The listing builds one solid part. Answer for the finished solid, in the listing's coordinates (mm). Round coordinates to 2 decimals unless told otherwise and drop trailing zeros. Write each loop counter-clockwise with the first axis right and the second up, starting at its lowest first coordinate (ties: lowest second). Pieces come first, ordered by that corner, then holes.
from build123d import *

# Parameters (mm, degrees)
SKETCH1_R           = 5.2
SKETCH1_R_2         = 10
BOSS_EXTRUDE1_DEPTH = 6
BOSS_EXTRUDE2_DEPTH = 6
BOSS_EXTRUDE4_DEPTH = 6


with BuildPart() as part:
    # Sketch1 → Boss-Extrude1 (new body)
    with BuildSketch(Plane(origin=(0, 0, 0), x_dir=(1, 0, 0), z_dir=(0, 1, 0))):
        with BuildLine():
            Line((-6.2, 0), (0, 95))
            Line((0, 95), (6.2, 0))
            Line((6.2, 0), (10.853330552, -28.209688314))
            ThreePointArc((10.853330552, -28.209688314), (0, -41), (-10.853330552, -28.209688314))
            Line((-10.853330552, -28.209688314), (-6.2, 0))
        make_face()
        with Locations(Location((0, 0, 0), (0, 0, 270))):
            Circle(SKETCH1_R, mode=Mode.SUBTRACT)
        with Locations(Location((0, -30, 0), (0, 0, 270))):
            Circle(SKETCH1_R_2, mode=Mode.SUBTRACT)
        with BuildLine():
            Line((-9.120824245, -23.850970395), (-5.618811795, -2.620868943))
            ThreePointArc((-5.618811795, -2.620868943), (0, -6.2), (5.618811795, -2.620868943))
            Line((5.618811795, -2.620868943), (9.120824245, -23.850970395))
            ThreePointArc((9.120824245, -23.850970395), (0, -19), (-9.120824245, -23.850970395))
        make_face(mode=Mode.SUBTRACT)
        with BuildLine():
            Line((-4.954626817, 3.727153486), (0, 79.644822449))
            Line((0, 79.644822449), (4.954626817, 3.727153486))
            ThreePointArc((4.954626817, 3.727153486), (0, 6.2), (-4.954626817, 3.727153486))
        make_face(mode=Mode.SUBTRACT)
    extrude(amount=BOSS_EXTRUDE1_DEPTH)

    # Sketch3 → Boss-Extrude2 (add)
    with BuildSketch(Plane(origin=(0, 0, 0), x_dir=(1, 0, 0), z_dir=(0, 1, 0))):
        with BuildLine():
            Line((4.841629208, 13.136157224), (4.913448664, 12.035697829))
            ThreePointArc((4.913448664, 12.035697829), (0, 13), (-4.913448664, 12.035697829))
            Line((-4.913448664, 12.035697829), (-4.841629208, 13.136157224))
            ThreePointArc((-4.841629208, 13.136157224), (0, 14), (4.841629208, 13.136157224))
        make_face()
        with BuildLine():
            Line((4.426036681, 19.504107242), (4.494123165, 18.460846594))
            ThreePointArc((4.494123165, 18.460846594), (0, 19), (-4.494123165, 18.460846594))
            Line((-4.494123165, 18.460846594), (-4.426036681, 19.504107242))
            ThreePointArc((-4.426036681, 19.504107242), (0, 20), (4.426036681, 19.504107242))
        make_face()
        with BuildLine():
            Line((4.022524974, 25.686947908), (4.089332805, 24.663279531))
            ThreePointArc((4.089332805, 24.663279531), (0, 25), (-4.089332805, 24.663279531))
            Line((-4.089332805, 24.663279531), (-4.022524974, 25.686947908))
            ThreePointArc((-4.022524974, 25.686947908), (0, 26), (4.022524974, 25.686947908))
        make_face()
        with BuildLine():
            Line((3.623950699, 31.794134386), (3.690163565, 30.779582402))
            ThreePointArc((3.690163565, 30.779582402), (0, 31), (-3.690163565, 30.779582402))
            Line((-3.690163565, 30.779582402), (-3.623950699, 31.794134386))
            ThreePointArc((-3.623950699, 31.794134386), (0, 32), (3.623950699, 31.794134386))
        make_face()
        with BuildLine():
            Line((3.227899864, 37.862655249), (3.293786636, 36.853099864))
            ThreePointArc((3.293786636, 36.853099864), (0, 37), (-3.293786636, 36.853099864))
            Line((-3.293786636, 36.853099864), (-3.227899864, 37.862655249))
            ThreePointArc((-3.227899864, 37.862655249), (0, 38), (3.227899864, 37.862655249))
        make_face()
        with BuildLine():
            ThreePointArc((2.899005539, 42.902165061), (0, 43), (-2.899005539, 42.902165061))
            Line((-2.899005539, 42.902165061), (-2.833317095, 43.908681536))
            ThreePointArc((-2.833317095, 43.908681536), (0, 44), (2.833317095, 43.908681536))
            Line((2.833317095, 43.908681536), (2.899005539, 42.902165061))
        make_face()
        with BuildLine():
            ThreePointArc((2.505223913, 48.935915779), (0, 49), (-2.505223913, 48.935915779))
            Line((-2.505223913, 48.935915779), (-2.439665173, 49.94044487))
            ThreePointArc((-2.439665173, 49.94044487), (0, 50), (2.439665173, 49.94044487))
            Line((2.439665173, 49.94044487), (2.505223913, 48.935915779))
        make_face()
        with BuildLine():
            ThreePointArc((2.112110327, 54.959430401), (0, 55), (-2.112110327, 54.959430401))
            Line((-2.112110327, 54.959430401), (-2.046641092, 55.962588041))
            ThreePointArc((-2.046641092, 55.962588041), (0, 56), (2.046641092, 55.962588041))
            Line((2.046641092, 55.962588041), (2.112110327, 54.959430401))
        make_face()
        with BuildLine():
            ThreePointArc((1.719465589, 60.97576107), (0, 61), (-1.719465589, 60.97576107))
            Line((-1.719465589, 60.97576107), (-1.654060735, 61.977932227))
            ThreePointArc((-1.654060735, 61.977932227), (0, 62), (1.654060735, 61.977932227))
            Line((1.654060735, 61.977932227), (1.719465589, 60.97576107))
        make_face()
        with BuildLine():
            ThreePointArc((1.327162667, 66.986854227), (0, 67), (-1.327162667, 66.986854227))
            Line((-1.327162667, 66.986854227), (-1.261805677, 67.988291981))
            ThreePointArc((-1.261805677, 67.988291981), (0, 68), (1.261805677, 67.988291981))
            Line((1.261805677, 67.988291981), (1.327162667, 66.986854227))
        make_face()
        with BuildLine():
            Line((-7.629550902, -11.738396528), (-7.450533577, -10.653147395))
            ThreePointArc((-7.450533577, -10.653147395), (0, -13), (7.450533577, -10.653147395))
            Line((7.450533577, -10.653147395), (7.629550902, -11.738396528))
            ThreePointArc((7.629550902, -11.738396528), (0, -14), (-7.629550902, -11.738396528))
        make_face()
        with BuildLine():
            Line((-8.666516131, -18.024746826), (-8.496550368, -16.994370593))
            ThreePointArc((-8.496550368, -16.994370593), (0, -19), (8.496550368, -16.994370593))
            Line((8.496550368, -16.994370593), (8.666516131, -18.024746826))
            ThreePointArc((8.666516131, -18.024746826), (0, -20), (-8.666516131, -18.024746826))
        make_face()
        with BuildLine():
            ThreePointArc((-8.308002125, -23.579166667), (-8.614654406, -23.996856701), (-8.900326734, -24.429166667))
            ThreePointArc((-8.900326734, -24.429166667), (0, -26), (8.900326734, -24.429166667))
            ThreePointArc((8.900326734, -24.429166667), (8.614654406, -23.996856701), (8.308002125, -23.579166667))
            ThreePointArc((8.308002125, -23.579166667), (0, -25), (-8.308002125, -23.579166667))
        make_face()
        with BuildLine():
            ThreePointArc((-10.467866671, -29.179166667), (0, -31), (10.467866671, -29.179166667))
            ThreePointArc((10.467866671, -29.179166667), (10.495821222, -29.703795885), (10.497498875, -30.229166667))
            ThreePointArc((10.497498875, -30.229166667), (0, -32), (-10.497498875, -30.229166667))
            ThreePointArc((-10.497498875, -30.229166667), (-10.495821222, -29.703795885), (-10.467866671, -29.179166667))
        make_face()
        with BuildLine():
            ThreePointArc((-8.631313108, -35.979166667), (0, -37), (8.631313108, -35.979166667))
            ThreePointArc((8.631313108, -35.979166667), (8.147195247, -36.6236855), (7.61506069, -37.229166667))
            ThreePointArc((7.61506069, -37.229166667), (0, -38), (-7.61506069, -37.229166667))
            ThreePointArc((-7.61506069, -37.229166667), (-8.147195247, -36.6236855), (-8.631313108, -35.979166667))
        make_face()
    extrude(amount=BOSS_EXTRUDE2_DEPTH)

    # Sketch5 → Boss-Extrude4 (add)
    with BuildSketch(Plane(origin=(0, 0, 0), x_dir=(1, 0, 0), z_dir=(0, 1, 0))):
        with BuildLine():
            Line((14.142215569, 53.100289487), (16, 50))
            ThreePointArc((16, 50), (15.802513368, 51.654776335), (15.221146562, 53.216601654))
            ThreePointArc((15.221146562, 53.216601654), (14.136998404, 54.76748473), (12.678547514, 55.973111763))
            ThreePointArc((12.678547514, 55.973111763), (10.40739911, 56.882764317), (7.962047997, 56.959189304))
            ThreePointArc((7.962047997, 56.959189304), (7.45389818, 56.86653646), (6.953920906, 56.73683098))
            ThreePointArc((6.953920906, 56.73683098), (5.366056739, 56.038714585), (3.997401273, 54.973134308))
            ThreePointArc((3.997401273, 54.973134308), (3.646986673, 54.596241795), (3.325075946, 54.194729849))
            ThreePointArc((3.325075946, 54.194729849), (2.72869668, 53.241749875), (2.291814027, 52.205905965))
            Line((2.291814027, 52.205905965), (2.435778417, 50))
            Line((2.435778417, 50), (2.936842105, 50))
            ThreePointArc((2.936842105, 50), (7.360037623, 55.813178764), (14.142215569, 53.100289487))
        make_face()
        with BuildLine():
            ThreePointArc((6.953920906, 56.73683098), (7.45389818, 56.86653646), (7.962047997, 56.959189304))
            Line((7.962047997, 56.959189304), (1.095242719, 70.540466335))
            Line((1.095242719, 70.540466335), (1.261318946, 67.995749955))
            Line((1.261318946, 67.995749955), (6.953920906, 56.73683098))
        make_face()
        with BuildLine():
            ThreePointArc((12.678547514, 55.973111763), (14.136998404, 54.76748473), (15.221146562, 53.216601654))
            Line((15.221146562, 53.216601654), (0.337667462, 82.148474304))
            Line((0.337667462, 82.148474304), (0.501063689, 79.644822449))
            Line((0.501063689, 79.644822449), (12.678547514, 55.973111763))
        make_face()
        with BuildLine():
            Line((2.045589816, 55.978696296), (2.291814027, 52.205905965))
            ThreePointArc((2.291814027, 52.205905965), (2.72869668, 53.241749875), (3.325075946, 54.194729849))
            Line((3.325075946, 54.194729849), (2.045589816, 55.978696296))
        make_face()
    boss_extrude4 = extrude(amount=BOSS_EXTRUDE4_DEPTH)

    # Mirror1: Boss-Extrude4 across plane
    add(boss_extrude4.mirror(Plane(origin=(0, 0, 0), x_dir=(0, 0, 1), z_dir=(1, 0, 0))))


solid = part.part
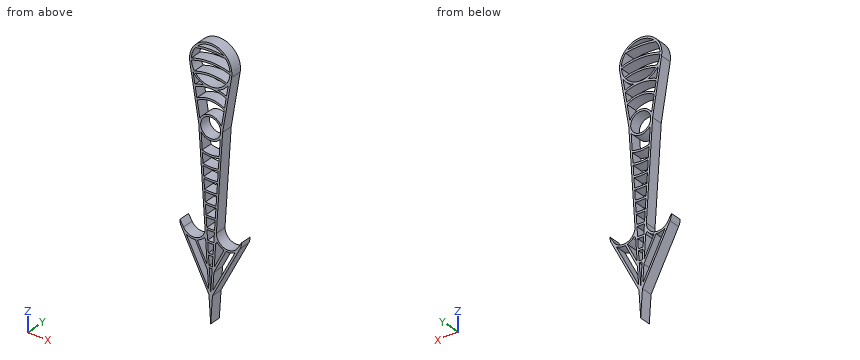
1. Given pin 1 (12 mm diameter, centred on x = -10, z = -2.5, fed in from +Y); pin 2 (2 mm diameter, centred on x = 4.5, y = 4.5, fed in from +Z); pin 3 (3 mm diameter, centred on x = -7, y = 1.5, fed in from +Z); pin 4 (1 mm diameter, centred on y = 2.5, z = 18, fed in from +X), each flat-ended and moving along its own axis, determine where each tip first touches the part or whether it passes through.
Geometry says:
pin 1: stops at y = 6
pin 2: stops at z = 40.43
pin 3: stops at z = 39.53
pin 4: stops at x = 9.25
2. Straight lines are drawn through the part: line 1 along X through (y, z) = (1.3, 0); line 2 along X through (y, z) = (1.7, -34.5); line 3 along X through (y, z) = (1.5, -86.5). For each, find the intervals that lie inside material, in ascending order.
Geometry says:
line 1: x = -6.2 to -5.2, 5.2 to 6.2
line 2: x = -3.95 to -2.95, 2.95 to 3.95
line 3: x = -0.55 to 0.55
3. Section A-A on z = -17 is taken. Determine the outline of the cut face in (x, y).
Geometry says:
outline: (-5.09, 0) - (-4.09, 0) - (-4.09, 6) - (-5.09, 6) - close; (4.09, 0) - (5.09, 0) - (5.09, 6) - (4.09, 6) - close
4. Section B-B on y = 4.8 is taken. Give the number of separate pieces and of enclosed holes in the cut face, plus the area to 3 significant figures.
Geometry says:
separate pieces: 1
enclosed holes: 24
area: 566 mm2
